Could you check a few things on this model? Use its own coordinates, in mm. Face numbers are marked on the shaded views. Give positions to 0.01 mm unless a question says otherwise; leave off trailing zeros. Write each loop counter-clockwise with the first axis right and the second up, starting at its lowest first coordinate (ties: lowest second). Pieces come first, ordered by that corner, then holes. Notation, with made-up numbers: (4.5, 79.25) -> (62.5, 79.25) arc R34 ccw to (62.5, 112.25) -> close; hole circle Ø6 at (33, 79). An arc over 180 degrees is marked (long way). One line per question, with ' | ' between items.
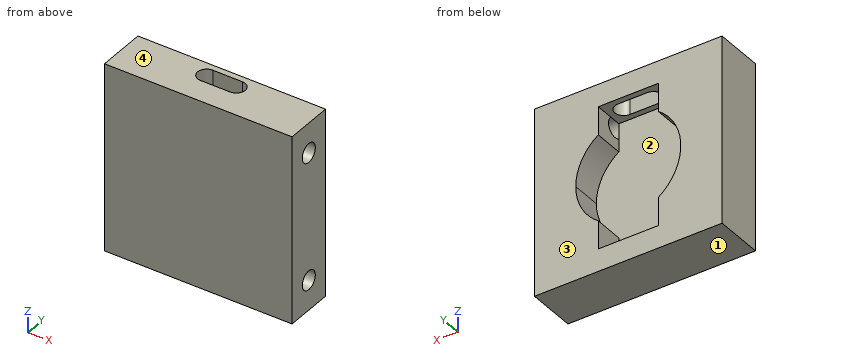
from build123d import *

# Parameters (mm, degrees)
SKETCH1_W                       = 50
SKETCH1_H                       = 50
BOSS_EXTRUDE1_DEPTH             = 13
BOSS_EXTRUDE2_DEPTH             = 5
F_8_0_199_DIAMETER_HOLE1_D      = 5.0546
F_8_0_199_DIAMETER_HOLE1_DEPTH  = 17
F_12_START                      = 19
F_12_0_189_DIAMETER_SLOT1_DEPTH = 6


# Read off the part's stored shape, not the designer's step: #12 (0.189) Diameter Slot1
with BuildPart() as part:
    # Sketch1 → Boss-Extrude1 (new body)
    with BuildSketch(Plane(origin=(0, 0, 0), x_dir=(1, 0, 0), z_dir=(0, 1, 0))):
        Rectangle(SKETCH1_W, SKETCH1_H)
        with BuildLine():
            Line((-8, 19), (8, 19))
            Line((8, 19), (8, 11.489125293))
            ThreePointArc((8, 11.489125293), (12.409673646, 6.480740698), (14, 0))
            ThreePointArc((14, 0), (12.409673646, -6.480740698), (8, -11.489125293))
            Line((8, -11.489125293), (8, -19))
            Line((8, -19), (-8, -19))
            Line((-8, -19), (-8, -11.489125293))
            ThreePointArc((-8, -11.489125293), (-14, 0), (-8, 11.489125293))
            Line((-8, 11.489125293), (-8, 19))
        make_face(mode=Mode.SUBTRACT)
    extrude(amount=BOSS_EXTRUDE1_DEPTH)

    # Sketch1<3> → Boss-Extrude2 (add)
    with BuildSketch(Plane(origin=(0, 0, 0), x_dir=(1, 0, 0), z_dir=(0, 1, 0))):
        with BuildLine():
            Line((8, -19), (8, -11.489125293))
            ThreePointArc((8, -11.489125293), (0, -14), (-8, -11.489125293))
            Line((-8, -11.489125293), (-8, -19))
            Line((-8, -19), (8, -19))
        make_face()
        with BuildLine():
            Line((8, -11.489125293), (8, 11.489125293))
            ThreePointArc((8, 11.489125293), (0, 14), (-8, 11.489125293))
            Line((-8, 11.489125293), (-8, -11.489125293))
            ThreePointArc((-8, -11.489125293), (0, -14), (8, -11.489125293))
        make_face()
        with BuildLine():
            Line((-8, -11.489125293), (-8, 11.489125293))
            ThreePointArc((-8, 11.489125293), (-14, 0), (-8, -11.489125293))
        make_face()
        with BuildLine():
            Line((8, 11.489125293), (8, 19))
            Line((8, 19), (-8, 19))
            Line((-8, 19), (-8, 11.489125293))
            ThreePointArc((-8, 11.489125293), (0, 14), (8, 11.489125293))
        make_face()
        with BuildLine():
            ThreePointArc((14, 0), (12.409673646, 6.480740698), (8, 11.489125293))
            Line((8, 11.489125293), (8, -11.489125293))
            ThreePointArc((8, -11.489125293), (12.409673646, -6.480740698), (14, 0))
        make_face()
    extrude(amount=BOSS_EXTRUDE2_DEPTH)

    # #8 (0.199) Diameter Hole1
    with Locations(Plane(origin=(25, 0, 0), x_dir=(0, 0, -1), z_dir=(1, 0, 0))):
        with Locations((-17, 6.5), (17, 6.5)):
            Hole(F_8_0_199_DIAMETER_HOLE1_D / 2, depth=F_8_0_199_DIAMETER_HOLE1_DEPTH)

    # #12 (0.189) Diameter Slot1 outline → #12 (0.189) Diameter Slot1 (cut)
    with BuildSketch(Plane.XY.offset(F_12_START)):
        with BuildLine():
            Line((-3.9497, 6.5997), (3.9497, 6.5997))
            ThreePointArc((3.9497, 6.5997), (6.35, 9), (3.9497, 11.4003))
            Line((3.9497, 11.4003), (-3.9497, 11.4003))
            ThreePointArc((-3.9497, 11.4003), (-6.35, 9), (-3.9497, 6.5997))
        make_face()
    extrude(amount=F_12_0_189_DIAMETER_SLOT1_DEPTH, mode=Mode.SUBTRACT)


solid = part.part
Q1. If we mould it in two halves opening along Z, with no side actions, what happens to the marked faces 1, 2, 3 and 4? For each: +Z half, -Z half, draft (parallel to the pull), parting line (faces both ways), or undercut.
Answer below:
face 1: -Z half | face 2: undercut | face 3: draft | face 4: +Z half
Q2. Imagine slicing it at B-B on z = -18. Please give me the cut outline in (x, y).
Answer below:
outline: (-25, 0) -> (25, 0) -> (25, 4.18) -> (8, 4.18) -> (8, 5) -> (-8, 5) -> (-8, 13) -> (-25, 13) -> close; (8, 8.82) -> (25, 8.82) -> (25, 13) -> (8, 13) -> close
Q3. Imagine slicing it at D-D on z = -3.5. Please give me the cut outline in (x, y), and give its area (3 significant figures).
Answer below:
outline: (-25, 0) -> (25, 0) -> (25, 13) -> (13.56, 13) -> (13.56, 5) -> (-13.56, 5) -> (-13.56, 13) -> (-25, 13) -> close | area: 433 mm^2
Q4. If I drill on line 1 along Z through (x, y) = (16.75, 6.5); line 2 along Z through (x, y) = (12, 6.5); line 3 along Y through (x, z) = (15.75, 17), over which ranges is the centre line in solid material (lowest first)?
Answer below:
line 1: z = -25 to -19.53, -14.47 to 14.47, 19.53 to 25 | line 2: z = -25 to -19.53, -14.47 to -7.21, 7.21 to 14.47, 19.53 to 25 | line 3: y = 0 to 3.97, 9.03 to 13
Q5. Imagine slicing it at C-C on x = -10. Please give me the cut outline in (y, z), and give its area (3 significant figures).
Answer below:
outline: (0, -25) -> (13, -25) -> (13, -9.8) -> (5, -9.8) -> (5, 9.8) -> (13, 9.8) -> (13, 25) -> (0, 25) -> close | area: 493 mm^2
Q6. Imagine slicing it at A-A on z = 20.5. Please give me the cut outline in (x, y), and give its area (3 significant figures).
Answer below:
outline: (-25, 0) -> (25, 0) -> (25, 13) -> (-25, 13) -> close; hole (-3.95, 6.6) -> (3.95, 6.6) arc R2.4 ccw to (3.95, 11.4) -> (-3.95, 11.4) arc R2.4 ccw to start | area: 594 mm^2
